Geometry: final body of the model. Coordinates: model frame, mm. A direction names the side the tool comes from. Give positions to 0.01 mm unless a question says otherwise; leave off trailing zeros. Loops run counter-clockwise (first coordinate to the right, second up) from the corner with the lowest first, then second, coordinate; pieces in that order, holes last. Notation, with made-up numbers: M 83,-11 L 120,-11 A20 cw 120,-6 Z; hole C 24,23.25 d6. An arc over 180 degrees is marked long. One line per question, with ' | ' between items. Start each with the question number.
from build123d import *

# Parameters (mm, degrees)
SKETCH1_W                                       = 50
SKETCH1_H                                       = 8
BOSS_EXTRUDE1_DEPTH                             = 20
SKETCH2_R                                       = 3
CUT_EXTRUDE1_DEPTH                              = 17
CUT_EXTRUDE2_DEPTH                              = 4
SKETCH4_W                                       = 10
SKETCH4_H                                       = 15
BOSS_EXTRUDE2_DEPTH                             = 8
CSK_FOR_M4_FLAT_HEAD_MACHINE_SCREW1_D           = 4.5
CSK_FOR_M4_FLAT_HEAD_MACHINE_SCREW1_CSINK_D     = 9.4
CSK_FOR_M4_FLAT_HEAD_MACHINE_SCREW1_CSINK_ANGLE = 90


with BuildPart() as part:
    # Sketch1 → Boss-Extrude1 (new body)
    with BuildSketch(Plane.XY):
        with Locations((-25, -15.35)):
            Rectangle(SKETCH1_W, SKETCH1_H)
        with Locations((25, -15.35)):
            Rectangle(SKETCH1_W, SKETCH1_H)
        with BuildLine():
            Line((40, -6.35), (12.432745191, -6.35))
            add(Edge.make_bspline(
                [(0, -11.35), (7.972410052, -11.35), (12.432745191, -6.35)],
                knots=[1.570796327, 1.570796327, 1.570796327, 2.547844784, 2.547844784, 2.547844784], degree=2, weights=[1, 0.883026434, 1]))
            Line((0, -11.35), (50, -11.35))
            Line((50, -11.35), (41.339745962, -6.35))
            Line((41.339745962, -6.35), (40, -6.35))
        make_face()
    extrude(amount=BOSS_EXTRUDE1_DEPTH)

    # Sketch2 → Cut-Extrude1 (cut)
    with BuildSketch(Plane(origin=(0, -6.35, 0), x_dir=(1, 0, 0), z_dir=(0, 1, 0))):
        with Locations((35, -10)):
            Circle(SKETCH2_R)
        with Locations((20, -10)):
            Circle(SKETCH2_R)
    extrude(amount=-CUT_EXTRUDE1_DEPTH, mode=Mode.SUBTRACT)

    # Sketch3 → Cut-Extrude2 (cut)
    with BuildSketch(Plane.XZ.offset(19.35)):
        with BuildLine():
            Line((20, 15.5), (35, 15.5))
            ThreePointArc((35, 15.5), (40.5, 10), (35, 4.5))
            Line((35, 4.5), (20, 4.5))
            ThreePointArc((20, 4.5), (14.5, 10), (20, 15.5))
        make_face()
    extrude(amount=-CUT_EXTRUDE2_DEPTH, mode=Mode.SUBTRACT)

    # Sketch4 → Boss-Extrude2 (add)
    with BuildSketch(Plane.XZ.offset(19.35)):
        with Locations((-45, 27.5)):
            Rectangle(SKETCH4_W, SKETCH4_H)
        with Locations((45, 27.5)):
            Rectangle(SKETCH4_W, SKETCH4_H)
        with Locations((-45, -7.5)):
            Rectangle(SKETCH4_W, SKETCH4_H)
        with Locations((45, -7.5)):
            Rectangle(SKETCH4_W, SKETCH4_H)
    extrude(amount=-BOSS_EXTRUDE2_DEPTH)

    # CSK for M4 Flat Head Machine Screw1 (through all)
    with Locations(Plane(origin=(0, -11.35, 0), x_dir=(1, 0, 0), z_dir=(0, 1, 0))):
        with Locations((-45, 10), (-45, -30), (45, -30), (45, 10)):
            CounterSinkHole(CSK_FOR_M4_FLAT_HEAD_MACHINE_SCREW1_D / 2, CSK_FOR_M4_FLAT_HEAD_MACHINE_SCREW1_CSINK_D / 2, counter_sink_angle=CSK_FOR_M4_FLAT_HEAD_MACHINE_SCREW1_CSINK_ANGLE)


solid = part.part
Q1. Section A-A, the plane x = -45. Output: boundary loops of the cut face in (y, z).
Q2. Section B-B, the plane z = -4. Output: boundary loops of the cut face in (x, y).
Q3. Draft query along Z for faces 5 (the flat face through (45, -15, -15)), 6 (the cylindrical face through (40.5, -17.4, 10.1)), 7 (the conical face through (-44.486, -13.681, 32.313)), 8 (the flat face through (45, -11.35, -4)). Return one class per face: released by +Z, released by -Z, zero draft, split by the parting line, or undercut.
Q4. Section C-C, the plane x = 19. Output: boundary loops of the cut face in (y, z), plus the area to 3 significant figures.
Q5. Material intervals for L1, parallel to Z at x = -45, y = -15.35; L2, parallel to X at y = -14, z = -10; L3, parallel to X at y = -13, z = 10, sorted ascending.
Q6. Set-up query: faces 1 (the flat face through (-31, -11.35, 10)), 2 (the flat face through (40, -15, -8)), 3 (the flat face through (28, -15.35, 10)), 4 (the flat face through (40, -15, 27)). Return all of +Z, -Z, +X, -X, +Y, -Y with unobstructed straight access to the full face (end or side cutting, diameter ignored); none if empty.
Q7. Contact query for flat-ended pins moving along their axis: pin 1 (5.5 mm diameter, centred on x = 32.5, z = 11, fed in from -Y); pin 2 (2 mm diameter, centred on x = -32.5, y = -14, fed in from +Z); pin 3 (2 mm diameter, centred on x = 28, y = -17, fed in from -Z). Output: stop coordinate, or through.
Q8. Section D-D, the plane z = 10. Count the separate pieces of the cut face and the enclosed holes in it, plus the area to 3 significant figures.
Model answer:
1) outline: M -19.35,-15 L -11.35,-15 L -11.35,-14.7 L -13.8,-12.25 L -19.35,-12.25 Z; M -19.35,-7.75 L -13.8,-7.75 L -11.35,-5.3 L -11.35,25.3 L -13.8,27.75 L -19.35,27.75 Z; M -19.35,32.25 L -13.8,32.25 L -11.35,34.7 L -11.35,35 L -19.35,35 Z
2) outline: M -50,-19.35 L -40,-19.35 L -40,-11.35 L -50,-11.35 Z; M 40,-19.35 L 50,-19.35 L 50,-11.35 L 40,-11.35 Z
3) face 5: released by -Z | face 6: undercut | face 7: undercut | face 8: zero draft
4) outline: M -19.35,0 L -6.35,0 L -6.35,7.17 L -15.35,7.17 L -15.35,4.59 L -19.35,4.59 Z; M -19.35,15.41 L -15.35,15.41 L -15.35,12.83 L -6.35,12.83 L -6.35,20 L -19.35,20 Z | area: 166 mm^2
5) L1: z = -15 to -12.25, -7.75 to 27.75, 32.25 to 35 | L2: x = -50 to -47.25, -42.75 to -40, 40 to 42.75, 47.25 to 50 | L3: x = -50 to 17, 23 to 32, 38 to 50
6) face 1: +Z, -Z, -X, +Y | face 2: -Z, +Y, -Y | face 3: -Y | face 4: +Z, +Y, -Y
7) pin 1: stops at y = -15.35 | pin 2: stops at z = 20 | pin 3: stops at z = 0
8) separate pieces: 3 | enclosed holes: 0 | area: 773 mm^2
